Check sheet for the modelled part. Datum: model origin and axes. Units: mm. A direction names the side the tool comes from. Round coordinates to 2 decimals unless told otherwise and drop trailing zeros. Order: outer loops, then holes, each group sorted by start corner. A loop starts at its lowest first (then second) coordinate and runs counter-clockwise, first axis right, second up.
Q1. Cross-section at A-A on z = -63.5. Record the cut outline in (x, y).
Q2. Depth check by flat-ended pin: P1, Ø3, axis at x = 71.5, y = 3.5, coming from the +Z side; P2, Ø2, axis at y = 6, z = -109.5, coming from the +X side; P3, Ø2.5, axis at y = 3, z = -119.5, coming from the +X side (3 decimals). Enter the tip coordinate at first touch or a pass-through.
Q3. Scan lines: probe 1 along X at (y, z) = (1.75, -11); probe 2 along X at (y, z) = (2, -58.5); probe 3 along Z at (x, y) = (36, 3). Record each from-to range of solid material in increasing order.
Q4. Cross-section at B-B on z = -136. Record the cut outline in (x, y) (3 decimals).
Q5. Mould release check, pull along X, two halves, no side actions. Record for faces 4 (the flat face through (72, 4, -146.05)), 5 (the flat face through (70.04, 4, -4)), 6 (the flat face through (0, 4, -127)): +X half, -X half, draft (parallel to the pull), parting line (faces both ways), or undercut.
Q6. Set-up check for faces 1 (the flat face through (142.875, 4, -127)), 2 (the flat face through (108.14, 4, -12)), 3 (the flat face through (147.638, 4, -53)): record each of +Z, -Z, +X, -X, +Y, -Y from which the full face is reachable in a straight line by a thin tool's end or side.
from build123d import *

# Parameters (mm, degrees)
BOSS_EXTRUDE1_DEPTH          = 8.382
CUT_EXTRUDE2_DEPTH           = 208.840544241
F_5_8_0_625_DIAMETER_HOLE1_D = 15.875
FILLET1_R                    = 1.27


with BuildPart() as part:
    # Sketch1 → Boss-Extrude1 (new body)
    with BuildSketch(Plane(origin=(0, 0, 0), x_dir=(1, 0, 0), z_dir=(0, 1, 0))):
        Polygon((0, 0), (142.875, 0), (147.6375, 0), (147.6375, 107.95), (142.875, 107.95), (142.875, 146.05), (0, 146.05), (0, 107.95), (-4.7625, 107.95), (-4.7625, 0), align=None)
    extrude(amount=BOSS_EXTRUDE1_DEPTH)

    # Sketch10 → Cut-Extrude2 (cut, through all)
    with BuildSketch(Plane(origin=(0, 8.382, 0), x_dir=(1, 0, 0), z_dir=(0, 1, 0))):
        Polygon((70.0405, 9.2075), (68.199, 9.2075), (68.199, 6.6675), (70.0405, 6.6675), (70.0405, 0), (72.8345, 0), (72.8345, 6.6675), (74.676, 6.6675), (74.676, 9.2075), (72.8345, 9.2075), (72.8345, 15.875), (70.0405, 15.875), align=None)
        Polygon((108.1405, 15.875), (110.9345, 15.875), (110.9345, 9.2075), (112.776, 9.2075), (112.776, 6.6675), (110.9345, 6.6675), (110.9345, 0), (108.1405, 0), (108.1405, 6.6675), (106.299, 6.6675), (106.299, 9.2075), (108.1405, 9.2075), align=None)
        Polygon((34.7345, 15.875), (34.7345, 9.2075), (36.576, 9.2075), (36.576, 6.6675), (34.7345, 6.6675), (34.7345, 0), (31.9405, 0), (31.9405, 6.6675), (30.099, 6.6675), (30.099, 9.2075), (31.9405, 9.2075), (31.9405, 15.875), align=None)
    extrude(amount=-CUT_EXTRUDE2_DEPTH, mode=Mode.SUBTRACT)

    # 5/8 (0.625) Diameter Hole1 (through all)
    with Locations(Plane(origin=(0, 0, 0), x_dir=(-1, 0, 0), z_dir=(0, -1, 0))):
        with Locations((-71.4375, 58.7375)):
            Hole(F_5_8_0_625_DIAMETER_HOLE1_D / 2)

    # Fillet1
    fillet1_edges = [part.edges().sort_by_distance(p)[0] for p in [
        (34.7345, 4.191, 0),
        (31.9405, 4.191, 0),
        (-4.7625, 4.191, 0),
        (-4.7625, 4.191, -107.95),
        (0, 4.191, -107.95),
        (0, 4.191, -146.05),
        (142.875, 4.191, -146.05),
        (142.875, 4.191, -107.95),
        (147.6375, 4.191, -107.95),
        (147.6375, 4.191, 0),
        (72.8345, 4.191, 0),
        (70.0405, 4.191, 0),
        (110.9345, 4.191, 0),
        (108.1405, 4.191, 0),
    ]]
    fillet(fillet1_edges, radius=FILLET1_R)


solid = part.part
Results found:
1. outline: (-4.76, 0) - (65.09, 0) - (65.09, 8.38) - (-4.76, 8.38) - close; (77.79, 0) - (147.64, 0) - (147.64, 8.38) - (77.79, 8.38) - close
2. P1: stops at z = -0.64
2. P2: stops at x = 143.1
2. P3: stops at x = 142.875
3. probe 1: x = -4.76 to 31.94, 34.73 to 70.04, 72.83 to 108.14, 110.93 to 147.64
3. probe 2: x = -4.76 to 63.5, 79.37 to 147.64
3. probe 3: z = -146.05 to -9.21, -6.67 to 0
4. outline: (0, 0) - (142.875, 0) - (142.875, 8.382) - (0, 8.382) - close
5. face 4: draft
5. face 5: undercut
5. face 6: -X half
6. face 1: -Z, +X, +Y, -Y
6. face 2: +Z, +Y, -Y
6. face 3: +Z, -Z, +X, +Y, -Y
